Study the drawing (mm; zero at the part's minimum x, y, z) and answer. A direction names the side the tool comes from. Give positions to 0.01 mm unless a question says otherwise; leave off trailing zeros. Loops run counter-clockwise (first coordinate to the right, second up) from the corner with the lowest first, then second, coordinate; pieces in that order, holes last. Notation, with made-up numbers: (88, -22.75) - (119, -22.75) arc R37 cw to (119, 14.25) - close; hole circle Ø9 at (45.5, 76). An arc over 180 degrees is marked (long way). Write item = value, one per line. Start each with the question number.
1) Consider probe 1 along X at (y, z) = (2.8, 4.25) (1 decimal); probe 2 along Z at (x, y) = (1.5, 1.95) (1 decimal); probe 3 along X at (y, z) = (0.7, 10). Determine where each line is inside the solid, lowest interval first.
2) The part is cut by section C-C on x = 2.5. Write down the section's boundary in (y, z) (1 decimal).
3) Which of the six approach directions +Z, -Z, +X, -X, +Y, -Y give full straight-line access (tool end or side, diameter ignored) to the marked faces 4, 5, 6 and 7?
4) The mould has two halves that part along Z. Classify the marked faces 1, 2 and 3: +Z half, -Z half, draft (parallel to the pull), parting line (faces both ways), or undercut.
5) The part is cut by section B-B on z = 11.5. Write down the section's boundary in (x, y) (1 decimal).
6) Flat-ended cylindrical pins translate along their axes: P1, Ø1, axis at x = 19, z = 14, coming from the -Y side; P2, Ø1.6, axis at y = 1, z = 1.5, coming from the +X side (1 decimal); P3, Ø1, axis at x = 24, y = 1.5, coming from the +Z side; P4, Ø1, axis at y = 1.5, z = 2.5, coming from the -X side (1 decimal). Find the tip coordinate at first contact, or state that the pin passes through.
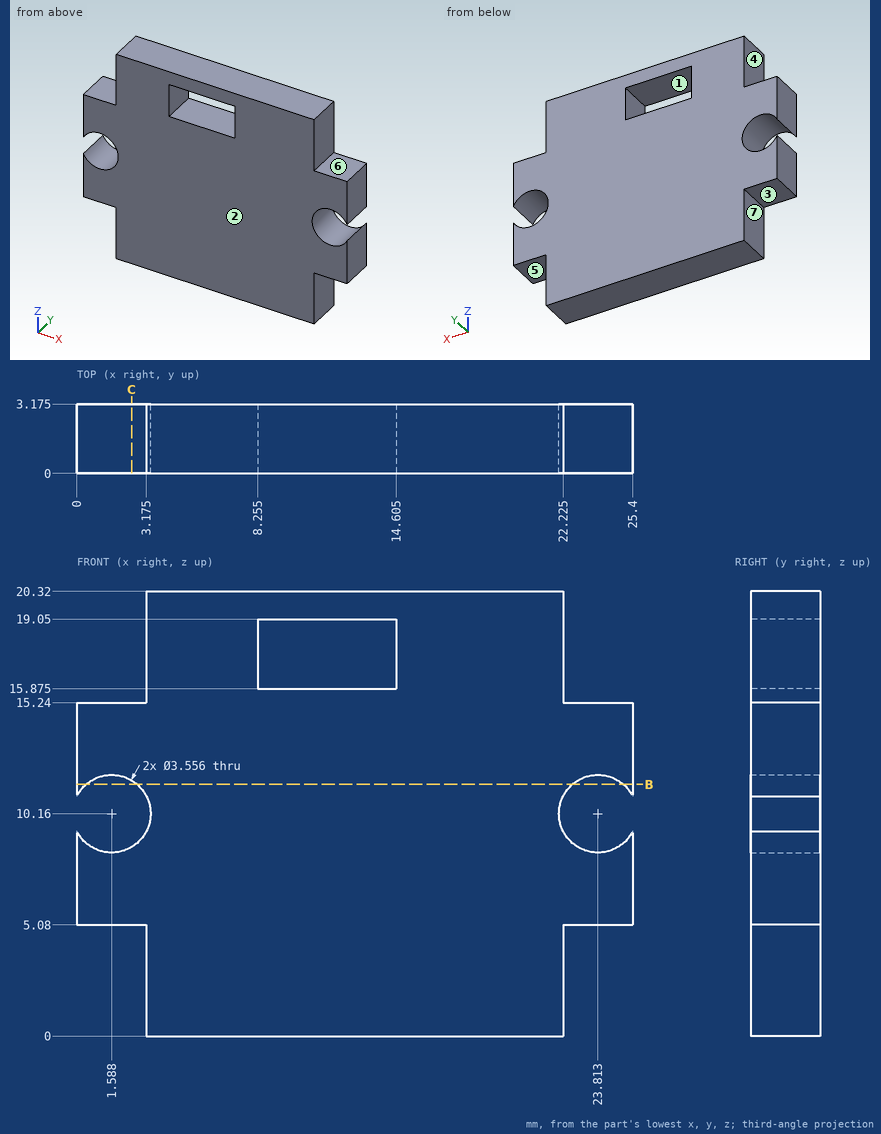
Answer below:
q1.probe_1 = 3.2 to 22.2
q1.probe_2 = 5.1 to 8.4, 11.9 to 15.2
q1.probe_3 = 3.36 to 22.04
q2.outline = (0, 5.1) - (3.2, 5.1) - (3.2, 8.6) - (0, 8.6) - close; (0, 11.7) - (3.2, 11.7) - (3.2, 15.2) - (0, 15.2) - close
q3.face_4 = +Z, -X, +Y, -Y
q3.face_5 = -Z, +X, +Y, -Y
q3.face_6 = +Z, +X, +Y, -Y
q3.face_7 = -Z, -X, +Y, -Y
q4.face_1 = undercut
q4.face_2 = draft
q4.face_3 = -Z half
q5.outline = (0, 0) - (0.4, 0) - (0.4, 3.2) - (0, 3.2) - close; (2.8, 0) - (22.6, 0) - (22.6, 3.2) - (2.8, 3.2) - close; (25, 0) - (25.4, 0) - (25.4, 3.2) - (25, 3.2) - close
q6.P1 = 0
q6.P2 = 22.2
q6.P3 = 15.24
q6.P4 = 3.2
